The model under review builds one solid part; all positions refer to its coordinate system, in mm. A direction names the side the tool comes from. Round coordinates to 2 decimals unless told otherwise and drop trailing zeros. Write each loop counter-clockwise with the first axis right and the second up, starting at its lowest first coordinate (ties: lowest second). Pieces come first, ordered by that corner, then holes. Notation, with made-up numbers: (0.5, 84.5) -> (37.5, 84.5) arc R24 ccw to (37.5, 115.5) -> close; hole circle Ø1 at (-26, -18). An arc over 180 degrees is marked (long way). Use CSV: the item, a comma, the result in double quotes. Start each with the question number.
1) Machinability: for faces 1 (the face through (-13.5, 0, 0)), 2 (the face through (11.4, -1.08, -4.88)), 3 (the face through (0, 4, 4)), which of the approach directions +Z, -Z, +X, -X, +Y, -Y give a long, thin tool a straight path to every point of the face, cutting with its end or side? Answer none if there is none.
2) Mouldability with a two-part tool opening along X and no side actions: class faces 4 (the face through (5, -2, -5)), 5 (the face through (10.56, 2.58, 4.05)), 6 (the face through (-6.21, -1.08, 4.88)) as released by +X, released by -X, zero draft, split by the parting line, or undercut.
3) Take a section at C-C, the plane x = 5.75. Give the boundary of the cut face in (y, z), then the cut area to 3 significant figures.
4) For pin 1 Ø8 at (x, z) = (9.5, -5.5) entering from -Y; pin 2 Ø1.5 at (x, z) = (1, 6.5) entering from -Y; pin 3 Ø2 at (y, z) = (3.5, 4) entering from -X, all flat-tipped, find the tip position at first contact; note any pin that passes through.
5) Wall thickness on probe 1 along X at (y, z) = (6.5, 3.75); probe 2 along X at (y, z) = (-2.75, 5); probe 3 along Z at (x, y) = (10.5, -3.5): over which ranges is each line inside the solid? List them lowest first. Write a range as [from, to].
Autodesk Inventor part; units mm, degrees
ref_plane "YZ Plane" through (0, 0, 0) normal (1, 0, 0) x (0, 1, 0)
ref_plane "XZ Plane" through (0, 0, 0) normal (0, 1, 0) x (-1, 0, 0)
ref_plane "XY Plane" through (0, 0, 0) normal (0, 0, 1) x (1, 0, 0)
sketch "Skizze1" plane through (0, 0, 0) normal (0, 0, 1) x (1, 0, 0)
  line L0 (0, 0) -> (0, 9)
  line L1 (3.5, 9) -> (3.5, 5)
  line L2 (3.5, 5) -> (10, 5)
  line L3 (10, 5) -> (10, 4.8)
  line L4 (10, 4.8) -> (11.1, 4.8)
  line L5 (11.1, 4.8) -> (11.1, 5)
  line L6 (11.1, 5) -> (11.7, 5)
  line L7 (11.9, 4.8) -> (11.9, 0)
  line L8 (11.9, 0) -> (0, 0)
  line L9 (11.7, 5) -> (11.9, 4.8)
  line L10 (0, 5) -> (-13.5, 5)
  line L11 (-13.5, 5) -> (-13.5, 0)
  line L12 (-13.5, 0) -> (0, 0)
  line L13 (3.5, 9) -> (0, 9)
  line L14 (5, 5) -> (5, 0) construction
  line L15 (3.5, 5.75) -> (5, 5.75)
  line L16 (5, 5.75) -> (5, 5)
  point P0 (11.9, 5)
  dimension "d0" = 9.6
  dimension "d1" = 10
  dimension "d2" = 1.1
  dimension "d3" = 0.2
  dimension "d4" = 0.2
  dimension "d5" = 0.6
  dimension "Gabel_FixationShaft_Contact_Thickness" = 3.5
  dimension "d29" = 10
  dimension "d30" = 13.5
  dimension "d37" = 18
  dimension "d39" = 5
  dimension "d40" = 1.5
  dimension "d41" = 11.5
revolve "Umdrehung1" add sketch "Skizze1" angle 360 about axis through (11.9, 0, 0) along (-1, 0, 0)
chamfer "Fase1" distance 0.2 angle 45 2 edges at (3.5, -9, 0) (0, -9, 0)
chamfer "Fase2" distance 1.25 angle 45 1 edges at (-13.5, -5, 0)
thread "Gewinde1"
properties part number "ParallelMecha_Gabel_Connection_JointShaft_Rillenkugellager" material "Edelstahl"
Values found:
1,face 1,"+Z, -Z, -X, +Y, -Y"
1,face 2,"+X"
1,face 3,"-X"
2,face 4,"released by +X"
2,face 5,"undercut"
2,face 6,"zero draft"
3,outline,"circle Ø10 at (0, 0)"
3,area,"78.5 mm²"
4,pin 1,"y = -4.77"
4,pin 2,"y = -6.92"
4,pin 3,"x = -12.93"
5,probe 1,"[0, 3.5]"
5,probe 2,"[0, 5]"
5,probe 3,"[-3.28, 3.28]"
